Check sheet for the modelled part. Datum: model origin and axes. Units: mm. Face numbers are marked on the shaded views. Round coordinates to 2 decimals unless told otherwise and drop trailing zeros. Write each loop counter-clockwise with the first axis right and the second up, starting at its lowest first coordinate (ties: lowest second). Pieces come first, ordered by that corner, then holes. Notation, with made-up numbers: (-26.5, 44.5) -> (-7.5, 44.5) arc R32 ccw to (-7.5, 80.5) -> close; hole circle Ø6 at (54.25, 75.5). An arc over 180 degrees is marked (long way). Answer as a JSON object with one key per item and string values. Group by question number.
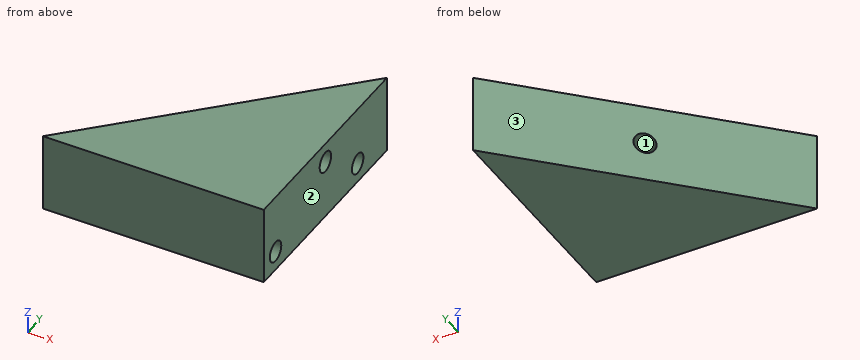
```python
from build123d import *

# Parameters (mm, degrees)
BOSS_EXTRUDE1_DEPTH = 15
SKETCH3_R           = 2
CUT_EXTRUDE1_DEPTH  = 20
SKETCH4_R           = 1.95
CUT_EXTRUDE2_DEPTH  = 5.4


with BuildPart() as part:
    # Sketch1 → Boss-Extrude1 (new body)
    with BuildSketch(Plane.XY):
        Polygon((0, 0), (42, 0), (42, 42), align=None)
    extrude(amount=BOSS_EXTRUDE1_DEPTH)

    # Sketch3 → Cut-Extrude1 (cut)
    with BuildSketch(Plane(origin=(0, 0, 0), x_dir=(0, 0, 1), z_dir=(-0.7071067811865477, 0.7071067811865475, 0))):
        with Locations(Location((7.5, 29.69848481, 0), (0, 0, 270))):
            Circle(SKETCH3_R)
    extrude(amount=-CUT_EXTRUDE1_DEPTH, mode=Mode.SUBTRACT)

    # Sketch4 → Cut-Extrude2 (cut)
    with BuildSketch(Plane(origin=(42, 0, 0), x_dir=(0, 0, -1), z_dir=(1, 0, 0))):
        with Locations((-11.25, 21)):
            Circle(SKETCH4_R)
        with Locations((-3.75, 4)):
            Circle(SKETCH4_R)
        with Locations((-3.75, 32)):
            Circle(SKETCH4_R)
    extrude(amount=-CUT_EXTRUDE2_DEPTH, mode=Mode.SUBTRACT)


solid = part.part
```
(1) Go/stop test with flat-tipped pins: pin 1 Ø5 at (y, z) = (4, 3.75) entering from -X; pin 2 Ø1.5 at (y, z) = (18.5, 10.5) entering from -X; pin 3 Ø3 at (y, z) = (21, 11.25) entering from -X. Record where each tip stops, or that it passes through.
(2) Scan lines: line 1 along Y through (x, z) = (39.85, 3.75); line 2 along Y through (x, z) = (39.6, 3.75); line 3 along X through (y, z) = (9.5, 13.5). Record each from-to range of solid material in increasing order.
(3) Section check D-D on y = 32. Record the cut outline in (x, z).
(4) Section check A-A on x = 38. Record the cut outline in (y, z).
(5) Release check for a two-part mould opening along Y. For the marked faces 1, 2 and 3 record: pulls with the +Y half, pulls with the -Y half, needs draft (parallel to the pull), parting line crosses it, or undercut.
(6) Section check B-B on y = 4. Record the cut outline in (x, z), then the cut area to 3 significant figures.
(7) Section check C-C on z = 11.25. Record the cut outline in (x, y).
Data:
{
 "1": {"pin 1": "stops at x = 1.5", "pin 2": "stops at x = 17.75", "pin 3": "stops at x = 19.5"},
 "2": {"line 1": "y = 0 to 2.05, 5.95 to 30.05, 33.95 to 39.85", "line 2": "y = 0 to 2.05, 5.95 to 30.05, 33.95 to 39.6", "line 3": "x = 9.5 to 42"},
 "3": {"outline": "(32, 0) -> (42, 0) -> (42, 1.8) -> (36.6, 1.8) -> (36.6, 5.7) -> (42, 5.7) -> (42, 15) -> (32, 15) -> close"},
 "4": {"outline": "(0, 0) -> (38, 0) -> (38, 15) -> (0, 15) -> close; hole circle Ø3.9 at (4, 3.75); hole circle Ø3.9 at (21, 11.25); hole circle Ø3.9 at (32, 3.75)"},
 "5": {"face 1": "undercut", "face 2": "needs draft", "face 3": "pulls with the +Y half"},
 "6": {"outline": "(4, 0) -> (42, 0) -> (42, 1.8) -> (36.6, 1.8) -> (36.6, 5.7) -> (42, 5.7) -> (42, 15) -> (4, 15) -> close", "area": "549 mm²"},
 "7": {"outline": "(0, 0) -> (42, 0) -> (42, 19.05) -> (36.6, 19.05) -> (36.6, 22.95) -> (42, 22.95) -> (42, 42) -> close"}
}
